from build123d import *

# Parameters (mm, degrees)
F3_D          = 8.2042
F5_R          = 1.9812
F6_DEPTH      = 15.876
F6_DEPTH_BACK = 15.876
F7_SIZE       = 0.508


with BuildPart() as f1:
    # F0 (on Right) → F1 (revolve)
    with BuildSketch(Plane.YZ):
        Polygon((0, 11.1827357164), (-101.6, 11.1827357164), (-101.6, -1.5172642836), (-54.6817518771, -1.5172642836), (-54.6817518771, 8.0077357164), (-15.1153696949, 8.0077357164), (3.175, 9.6079357164), (3.175, 14.3577357164), (0, 14.3577357164), align=None)
    revolve(axis=Axis((0, -78.1408759385, -1.5172642836), (0, 1, 0)))

    # F3 (through all)
    with Locations(Plane.XZ.offset(101.6)):
        with Locations((0, -1.5172642836)):
            Hole(F3_D / 2)

    # F5 (on face) → F6 (cut, two sides)
    with BuildSketch(Plane(origin=(0, 0, -1.5172642836), x_dir=(1, 0, 0), z_dir=(0, 0, -1))) as f6_sk:
        with Locations((0, 69.85)):
            Circle(F5_R)
    extrude(amount=-F6_DEPTH, mode=Mode.SUBTRACT)
    extrude(f6_sk.sketch, amount=F6_DEPTH_BACK, mode=Mode.SUBTRACT)

    # F7
    f7_edges = [f1.edges().sort_by_distance(p)[0] for p in [
        (0, -101.6, -14.217264),
    ]]
    chamfer(f7_edges, length=F7_SIZE)


solid = f1.part
Source: CAD feature listing. Evaluate the final solid. Frame: model axes, mm. A direction names the side the tool comes from. Round coordinates to 2 decimals unless told otherwise and drop trailing zeros. Loops run counter-clockwise (first coordinate to the right, second up) from the corner with the lowest first, then second, coordinate; pieces in that order, holes last.
Q1. Mould query, pull axis Y, two halves, no side actions, for faces 4 (the face through (-15.497, 1.565, -4.959)), 5 (the face through (11, 3.175, -5)), 6 (the face through (1.83, -69.09, 6.56)). Classes: pulls with the +Y half, pulls with the -Y half, needs draft (parallel to the pull), parting line crosses it, or undercut.
Q2. Section A-A, the plane x = 0. Return loops of the section in (y, z) (3 decimals).
Q3. Section B-B, the plane y = -69.85. Return loops of the section in (x, z).
Q4. First-contact query: P1, Ø4, axis at y = -19.5, z = 10, coming from the -X side; P2, Ø13, axis at x = 0, z = -1.52, coming from the -Y side; P3, Ø3, axis at y = -10, z = -1.5, coming from the -X side; P4, Ø1.5, axis at x = -6, y = -89, coming from the +Z side. Flat tips, straight axial feed; report the tip coordinate or a pass-through.
Q5. Section D-D, the plane x = 14.5. Return loops of the section in (y, z) (3 decimals).
Q6. Access query for faces 1 (the face through (1.83, -69.09, -9.6)), 2 (the face through (-7.728, -51.254, -11.596)), 3 (the face through (2.86, -34.62, 7.57)). Directions: +Z, -Z, +X, -X, +Y, -Y. A direction counts if a zero-diameter tool reaches every point of the face in a straight line with its end or side. Return the directions, or none.
Q7. Ray query, line 1 (Y direction, x = 0, z = -8.25); line 2 (Y direction, x = 3.5, z = 2.5); line 3 (X direction, y = -10.5, z = -8). Return the intervals inside material, ascending.
Q8. Section C-C, the plane y = -24. Return loops of the section in (x, z) (3 decimals).
Solutions:
1. face 4: needs draft
1. face 5: pulls with the +Y half
1. face 6: undercut
2. outline: (-101.6, -13.709) - (-101.092, -14.217) - (-71.831, -14.217) - (-71.831, -5.619) - (-101.6, -5.619) - close; (-101.6, 2.585) - (-71.831, 2.585) - (-71.831, 11.183) - (-101.092, 11.183) - (-101.6, 10.675) - close; (-67.869, -14.217) - (0, -14.217) - (0, -17.392) - (3.175, -17.392) - (3.175, -12.642) - (-15.115, -11.042) - (-54.682, -11.042) - (-54.682, -5.619) - (-67.869, -5.619) - close; (-67.869, 2.585) - (-54.682, 2.585) - (-54.682, 8.008) - (-15.115, 8.008) - (3.175, 9.608) - (3.175, 14.358) - (0, 14.358) - (0, 11.183) - (-67.869, 11.183) - close
3. outline: (-1.98, -14.06) - (-1.98, -5.11) arc R4.1 cw to (-1.98, 2.07) - (-1.98, 11.03) arc R12.7 ccw to start; (1.98, -14.06) arc R12.7 ccw to (1.98, 11.03) - (1.98, 2.07) arc R4.1 cw to (1.98, -5.11) - close
4. P1: stops at x = -8.41
4. P2: stops at y = -101.6
4. P3: stops at x = -12.7
4. P4: stops at z = 10.05
5. outline: (0, -7.98) - (3.175, -7.98) - (3.175, 4.945) - (0, 4.945) - close
6. face 1: +Z, -Z
6. face 2: -Y
6. face 3: +Y
7. line 1: y = -101.6 to -71.83, -67.87 to -54.68
7. line 2: y = -101.6 to -54.68
7. line 3: x = -10.92 to -7.52, 7.52 to 10.92
8. outline: circle Ø25.4 at (0, -1.517); hole circle Ø19.05 at (0, -1.517)
